Could you check a few things on this model? Use its own coordinates, in mm. A direction names the side the tool comes from. Round coordinates to 2 decimals unless told otherwise and drop trailing zeros. Write each loop counter-clockwise with the first axis right and the second up, starting at its lowest first coordinate (ties: lowest second). Pieces come first, ordered by that corner, then holes. Notation, with made-up numbers: (11.25, 3) - (63.25, 3) arc R14 ccw to (63.25, 20) - close; hole circle Ø2 at (22, -23). An arc over 180 degrees is marked (long way). Put each result on its own line as item: value.
from build123d import *

# Parameters (mm, degrees)
SKETCH1_W           = 20
SKETCH1_H           = 20
BOSS_EXTRUDE1_DEPTH = 20
SKETCH2_W           = 17.5
SKETCH2_H           = 17.5
CUT_EXTRUDE1_DEPTH  = 17.5
FILLET1_R           = 2.5


with BuildPart() as part:
    # Sketch1 → Boss-Extrude1 (new body)
    with BuildSketch(Plane(origin=(0, 20, 0), x_dir=(1, 0, 0), z_dir=(0, 1, 0))):
        with Locations((10, -10)):
            Rectangle(SKETCH1_W, SKETCH1_H)
    extrude(amount=-BOSS_EXTRUDE1_DEPTH)

    # Sketch2 → Cut-Extrude1 (cut)
    with BuildSketch(Plane(origin=(0, 0, 0), x_dir=(-1, 0, 0), z_dir=(0, 0, -1))):
        with Locations((-8.75, 8.75)):
            Rectangle(SKETCH2_W, SKETCH2_H)
    extrude(amount=-CUT_EXTRUDE1_DEPTH, mode=Mode.SUBTRACT)

    # Fillet1
    fillet1_edges = [part.edges().sort_by_distance(p)[0] for p in [
        (20, 20, 10),
        (10, 20, 20),
        (20, 10, 20),
    ]]
    fillet(fillet1_edges, radius=FILLET1_R)


solid = part.part
(1) For faces 1 (the face through (9, 9, 20)), 2 (the face through (9, 17.5, 9)), which set-ups out of +Z, -Z, +X, -X, +Y, -Y let a thin tool reach every point of the face, with its end or its side?
Values found:
face 1: +Z, +X, -X, +Y, -Y
face 2: -Z, -X, -Y
(2) Imagine slicing it at A-A, the plane x = 14. List the corners of the cut face in (y, z) for me.
Values found:
outline: (0, 17.5) - (17.5, 17.5) - (17.5, 0) - (20, 0) - (20, 17.5) arc R2.5 ccw to (17.5, 20) - (0, 20) - close
(3) Please list where this line runs through material, in increasing order: probe 1 along Z at (x, y) = (4.75, 15.5). Write a range as from..to.
Values found:
probe 1: z = 17.5..20
(4) I'm going to push flat-ended pins straight in: pin 1 (1 mm diameter, centred on x = 15, y = 12, fed in from -Z); pin 2 (9 mm diameter, centred on y = 11.5, z = 6.5, fed in from -X); pin 3 (9 mm diameter, centred on x = 7.5, z = 9, fed in from -Y). Where does each tip first touch, or does it pass through?
Values found:
pin 1: stops at z = 17.5
pin 2: stops at x = 17.5
pin 3: stops at y = 17.5
